from build123d import *

# Parameters (mm, degrees)
ESQUISSE1_W        = 1200
ESQUISSE1_H        = 1000
BOSS_EXTRU_1_DEPTH = 40
ESQUISSE2_W        = 250
ESQUISSE2_H        = 250
BOSS_EXTRU_2_DEPTH = 100


with BuildPart() as part:
    # Esquisse1 → Boss.-Extru.1 (new body)
    with BuildSketch(Plane(origin=(0, 0, 0), x_dir=(1, 0, 0), z_dir=(0, 1, 0))):
        Rectangle(ESQUISSE1_W, ESQUISSE1_H)
    extrude(amount=-BOSS_EXTRU_1_DEPTH)

    # Esquisse2 → Boss.-Extru.2 (add)
    with BuildSketch(Plane.XZ.offset(40)):
        Rectangle(ESQUISSE2_W, ESQUISSE2_H)
    extrude(amount=BOSS_EXTRU_2_DEPTH)


solid = part.part
CAD build for the part. Positions are in the model's coordinates, mm. A direction names the side the tool comes from. Coordinates: 2 decimals unless noted, no trailing zeros. Loops run counter-clockwise (first coordinate to the right, second up) from the corner with the lowest first, then second, coordinate; pieces in that order, holes last. Notation, with made-up numbers: (-32, 65) - (12, 65) arc R31 cw to (12, 91) - close; hole circle Ø4 at (87.25, 18). An arc over 180 degrees is marked (long way). Use one line per item in the form item = value. Start each with the question number.
1) Band-saw the part on C-C (y = -66). Give the cut face in (x, z).
2) Band-saw the part on B-B (x = -40.5). Give the cut face in (y, z), and give its area (3 significant figures).
3) Two-plate mould, pull along X, no slides. Class faces 1 (the face through (-600, -20, 7)), 2 (the face through (125, -89, -2)), 3 (the face through (-8, -20, -500)): +X half, -X half, draft (parallel to the pull), parting line (faces both ways), or undercut.
4) Tool access for faces 4 (the face through (-2, -89, 125)), 5 (the face through (-2, -89, -125)), 6 (the face through (-8, 0, -7)), 7 (the face through (-125, -89, -2)): list every direction of +Z, -Z, +X, -X, +Y, -Y with a clear straight run to the whole face (end or side of a thin tool).
5) Flat gauge pin, fed straight in: pin 1 (6 mm diameter, centred on x = 451.5, z = 113.5, fed in from -Y). Where does the tip first touch, or does it go through?
6) Band-saw the part on D-D (x = 488). Give the cut face in (y, z), and give its area (3 significant figures).
7) Drill centre lines: L1, parallel to Y at x = 315.5, z = 144.5; L2, parallel to X at y = -79, z = 90. Where is each one in solid material? Low to high. Write a range as from..to.
8) Band-saw the part on A-A (z = -106). Give the cut face in (x, y), and give its area (3 significant figures).
Check values:
q1.outline = (-125, -125) - (125, -125) - (125, 125) - (-125, 125) - close
q2.outline = (-140, -125) - (-40, -125) - (-40, -500) - (0, -500) - (0, 500) - (-40, 500) - (-40, 125) - (-140, 125) - close
q2.area = 65,000 mm2
q3.face_1 = -X half
q3.face_2 = +X half
q3.face_3 = draft
q4.face_4 = +Z, +X, -X, -Y
q4.face_5 = -Z, +X, -X, -Y
q4.face_6 = +Z, -Z, +X, -X, +Y
q4.face_7 = +Z, -Z, -X, -Y
q5.pin_1 = -40
q6.outline = (-40, -500) - (0, -500) - (0, 500) - (-40, 500) - close
q6.area = 40,000 mm2
q7.L1 = -40..0
q7.L2 = -125..125
q8.outline = (-600, -40) - (-125, -40) - (-125, -140) - (125, -140) - (125, -40) - (600, -40) - (600, 0) - (-600, 0) - close
q8.area = 73,000 mm2
